The drawing under review shows one solid part. Ordinate dimensions are in mm from its lowest x, y, z. A direction names the side the tool comes from. Coordinates: 2 decimals unless noted, no trailing zeros. Order: outer loops, then holes, each group sorted by start corner. A loop starts at its lowest first (then second) coordinate and runs counter-clockwise, first axis right, second up. Notation, with made-up numbers: (34, -25) -> (59, -25) arc R28 cw to (59, 0) -> close; hole circle Ø8 at (17.25, 61). An arc over 180 degrees is marked (long way). Put each result on its own line as item: value.
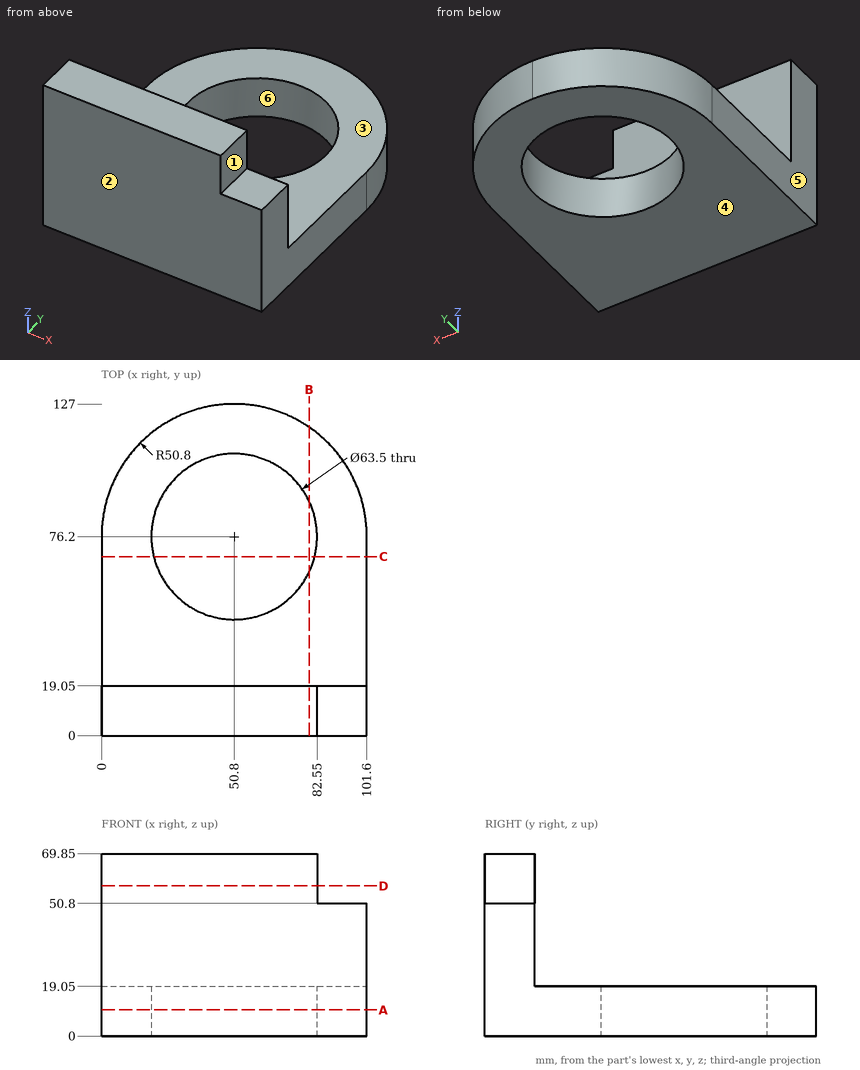
Item 1: For line 1 (Y direction, x = 50.8, z = 4.5); line 2 (Y direction, x = 10, z = 53.5), list the stretches that pass through material, from the lowest coordinate up. Write a range as from..to.
Answers below:
line 1: 0..44.45, 107.95..127
line 2: 0..19.05
Item 2: For pin 1 Ø15 at (y, z) = (13, 56) entering from +X; pin 2 Ø12 at (x, y) = (18.5, 83) entering from +Z; pin 3 Ø6 at (x, z) = (52.5, 47.5) entering from +Y; pin 4 Ø15 at (x, y) = (97, 13) entering from +Z, all flat-tipped, find the tip position at first contact; note any pin that passes through.
Answers below:
pin 1: x = 101.6
pin 2: z = 19.05
pin 3: y = 19.05
pin 4: z = 50.8
Item 3: For the marked faces 1, 2 and 3, list the 3-axis set-ups (+Z, -Z, +X, -X, +Y, -Y) from which the entire face can be reached by the end or side of a thin tool; tool diameter is ignored.
Answers below:
face 1: +Z, +X, +Y, -Y
face 2: +Z, -Z, +X, -X, -Y
face 3: +Z, +X, -X, +Y
Item 4: Consider section D-D on z = 57.5. Write out the cut boundary in (x, y).
Answers below:
outline: (0, 0) -> (82.55, 0) -> (82.55, 19.05) -> (0, 19.05) -> close
Item 5: Consider section C-C on y = 68.5. Write out the cut boundary in (x, z).
Answers below:
outline: (0, 0) -> (20, 0) -> (20, 19.05) -> (0, 19.05) -> close; (81.6, 0) -> (101.6, 0) -> (101.6, 19.05) -> (81.6, 19.05) -> close
Item 6: Mouldability with a two-part tool opening along X and no side actions: class the marked faces 4, 5 and 6 as +X half, -X half, draft (parallel to the pull), parting line (faces both ways), or undercut.
Answers below:
face 4: draft
face 5: -X half
face 6: undercut
Item 7: Consider section A-A on z = 10. Write out the cut boundary in (x, y).
Answers below:
outline: (0, 0) -> (101.6, 0) -> (101.6, 76.2) arc R50.8 ccw to (50.8, 127) arc R50.8 ccw to (0, 76.2) -> close; hole circle Ø63.5 at (50.8, 76.2)
Item 8: Consider section B-B on x = 79.5. Write out the cut boundary in (y, z).
Answers below:
outline: (0, 0) -> (62.62, 0) -> (62.62, 19.05) -> (19.05, 19.05) -> (19.05, 69.85) -> (0, 69.85) -> close; (89.78, 0) -> (118.12, 0) -> (118.12, 19.05) -> (89.78, 19.05) -> close
